Part model, mm, in its own coordinate system. Give positions to 0.01 mm unless a question says otherwise; leave off trailing zeros. Put each result on its own line as item: value. Start each with the question number.
```python
from build123d import *

# Parameters (mm, degrees)
SKETCH1_W           = 80
SKETCH1_H           = 60
BOSS_EXTRUDE2_DEPTH = 2
SKETCH3_R           = 1
CUT_EXTRUDE2_DEPTH  = 2
FILLET2_R           = 5


with BuildPart() as part:
    # Sketch1 → Boss-Extrude2 (new body)
    with BuildSketch(Plane(origin=(0, 0, 0), x_dir=(1, 0, 0), z_dir=(0, 1, 0))):
        with Locations((0.468384075, -9.016393443)):
            Rectangle(SKETCH1_W, SKETCH1_H)
    extrude(amount=BOSS_EXTRUDE2_DEPTH)

    # Sketch3 → Cut-Extrude2 (cut)
    with BuildSketch(Plane(origin=(0, 2, 0), x_dir=(1, 0, 0), z_dir=(0, 1, 0))):
        with Locations(Location((-32.031615925, -1.016393443, 0), (0, 0, 270))):
            Circle(SKETCH3_R)
        with Locations(Location((-32.031615925, -17.016393443, 0), (0, 0, 270))):
            Circle(SKETCH3_R)
        with Locations(Location((32.968384075, -1.016393443, 0), (0, 0, 270))):
            Circle(SKETCH3_R)
        with Locations(Location((32.968384075, -17.016393443, 0), (0, 0, 270))):
            Circle(SKETCH3_R)
        with Locations(Location((0.468384075, -9.016393443, 0), (0, 0, 270))):
            Circle(SKETCH3_R)
    extrude(amount=-CUT_EXTRUDE2_DEPTH, mode=Mode.SUBTRACT)

    # Fillet2
    fillet2_edges = [part.edges().sort_by_distance(p)[0] for p in [
        (-39.531615925, 1, -20.983606557),
        (40.468384075, 1, -20.983606557),
        (40.468384075, 1, 39.016393443),
        (-39.531615925, 1, 39.016393443),
    ]]
    fillet(fillet2_edges, radius=FILLET2_R)


solid = part.part
```
1) Pin check, flat tip, straight feed: pin 1 Ø1.2 at (x, z) = (-32.03, 17.02) entering from +Y. Stop position of the tip, or through.
2) Mould opens along X. For faces 1 (the cylindrical face through (33.812, 1.014, 1.554)), 2 (the flat face through (0, 2, 15)), 3 (the cylindrical face through (-38.11, 1.01, 37.51)), 4 (the cylindrical face through (-31.04, 1.01, 0.89)) say: +X half, -X half, draft (parallel to the pull), parting line (faces both ways), or undercut.
3) Wall check: L1, parallel to Z at x = 0.5, y = 0.45; L2, parallel to X at y = 1.8, z = 16.5; L3, parallel to X at y = 1.2, z = 9. Give the ranges that are in metal, low to high.
Evaluation:
1. pin 1: through
2. face 1: undercut
2. face 2: draft
2. face 3: -X half
2. face 4: undercut
3. L1: -20.98 to 8.02, 10.02 to 39.02
3. L2: -39.53 to -32.89, -31.18 to 32.11, 33.82 to 40.47
3. L3: -39.53 to -0.53, 1.47 to 40.47
